The model under review builds one solid part; all positions refer to its coordinate system, in mm. A direction names the side the tool comes from. Coordinates: 2 decimals unless noted, no trailing zeros. Loops run counter-clockwise (first coordinate to the right, second up) from the corner with the lowest first, then second, coordinate; pieces in that order, holes last. Notation, with made-up numbers: M -17,51.25 L -13,51.25 A21 cw -13,63.25 Z; hole C 40.25,53 d7. An arc over 180 degrees is marked long. One line per item, written item: value.
```python
from build123d import *

# Parameters (mm, degrees)
F0_W      = 99.06
F0_H      = 99.06
F1_DEPTH  = 4.445
F0_W_2    = 101.6
F0_H_2    = 101.6
F2_DEPTH  = 63.5
F5_R      = 14.2875
F7_DEPTH  = 25.4
F3_R      = 14.2875
F3_R_2    = 13.193858
F8_DEPTH  = 25.4
F4_R      = 14.2875
F4_R_2    = 14.425909
F9_DEPTH  = 25.4
F6_R      = 14.2875
F10_DEPTH = 25.4
F11_R     = 14.2875
F12_DEPTH = 25.4


with BuildPart() as f1:
    # F0 (on Top) → F1 (new body)
    with BuildSketch(Plane.XY):
        Rectangle(F0_W, F0_H)
    extrude(amount=F1_DEPTH)

    # F0 (on Top) → F2 (join)
    with BuildSketch(Plane.XY):
        Rectangle(F0_W_2, F0_H_2)
        Rectangle(F0_W, F0_H, mode=Mode.SUBTRACT)
    extrude(amount=F2_DEPTH)

    # F5 (on face) → F7 (cut)
    with BuildSketch(Plane.XZ.offset(50.8)):
        with Locations((-27.728472, 33.152512)):
            Circle(F5_R)
        with Locations((26.523072, 33.849479)):
            Circle(F5_R)
    extrude(amount=-F7_DEPTH, mode=Mode.SUBTRACT)

    # F3 (on face) → F8 (cut)
    with BuildSketch(Plane.YZ.offset(50.8)):
        with Locations((-27.133925, 33.572733)):
            Circle(F3_R)
        with Locations((24.041634, 33.572733)):
            Circle(F3_R_2)
    extrude(amount=-F8_DEPTH, mode=Mode.SUBTRACT)

    # F4 (on face) → F9 (cut)
    with BuildSketch(Plane(origin=(0, 50.8, 0), x_dir=(-1, 0, 0), z_dir=(0, 1, 0))):
        with Locations((-27.319755, 33.915631)):
            Circle(F4_R)
        with Locations((28.376452, 33.915631)):
            Circle(F4_R_2)
    extrude(amount=F9_DEPTH, mode=Mode.SUBTRACT)

    # F6 (on face) → F10 (cut)
    with BuildSketch(Plane(origin=(-50.8, 0, 0), x_dir=(0, -1, 0), z_dir=(-1, 0, 0))):
        with Locations((-24.966941, 34.00825)):
            Circle(F6_R)
        with Locations((27.751417, 33.17856)):
            Circle(F6_R)
    extrude(amount=-F10_DEPTH, mode=Mode.SUBTRACT)

    # F11 (on face) → F12 (cut)
    with BuildSketch(Plane(origin=(0, 50.8, 0), x_dir=(-1, 0, 0), z_dir=(0, 1, 0))):
        with Locations((-25.37245, 35.114542)):
            Circle(F11_R)
        with Locations((23.656343, 35.114542)):
            Circle(F11_R)
    extrude(amount=-F12_DEPTH, mode=Mode.SUBTRACT)


solid = f1.part
```
(1) To check wall thickness, follow L1, parallel to X at y = -14, z = 44; L2, parallel to Z at x = -29, y = 30.5 (3 decimals). State the ranges of each line that lie inside material, in increasing order. Write a range as [from, to].
Checks:
L1: [-50.8, -49.53], [49.53, 50.8]
L2: [0, 4.445]
(2) Add section C-C on x = 34. State the section outline as (y, z) points (3 decimals).
Checks:
outline: M -50.8,0 L 50.8,0 L 50.8,23.726 L 49.53,23.726 L 49.53,4.445 L -49.53,4.445 L -49.53,21.675 L -50.8,21.675 Z; M -50.8,46.024 L -49.53,46.024 L -49.53,63.5 L -50.8,63.5 Z; M 49.53,46.503 L 50.8,46.503 L 50.8,63.5 L 49.53,63.5 Z
(3) Add section A-A on z = 56. State the section outline as (x, y) points, then the cut area to 3 significant figures.
Checks:
outline: M -50.8,-50.8 L 50.8,-50.8 L 50.8,50.8 L -50.8,50.8 Z; hole M -49.53,-49.53 L 49.53,-49.53 L 49.53,49.53 L -49.53,49.53 Z
area: 510 mm^2
(4) Insertion check: pin 1 Ø3 at (x, y) = (-30, 24) entering from +Z (3 decimals). The pin has a flat end and moves straight along its axis. Give the tip position at first contact, or say it passes through.
Checks:
pin 1: z = 4.445
(5) Add section D-D on y = -21. State the section outline as (x, z) points (3 decimals).
Checks:
outline: M -50.8,0 L 50.8,0 L 50.8,20.669 L 49.53,20.669 L 49.53,4.445 L -49.53,4.445 L -49.53,20.587 L -50.8,20.587 Z; M -50.8,45.77 L -49.53,45.77 L -49.53,63.5 L -50.8,63.5 Z; M 49.53,46.477 L 50.8,46.477 L 50.8,63.5 L 49.53,63.5 Z
(6) Draft analysis for pull direction X (two halves, no side actions). For faces 1 (the face through (35.903, 50.174, 44.771)), 2 (the face through (-50.17, -34.34, 20.5)), 3 (the face through (50.8, -1, 31)), state which applies: pulls with the +X half, pulls with the -X half, needs draft (parallel to the pull), parting line crosses it, or undercut.
Checks:
face 1: undercut
face 2: needs draft
face 3: pulls with the +X half
(7) Add section B-B on y = -2. State the section outline as (x, z) points (3 decimals), then the cut area to 3 significant figures.
Checks:
outline: M -50.8,0 L 50.8,0 L 50.8,63.5 L 49.53,63.5 L 49.53,4.445 L -49.53,4.445 L -49.53,63.5 L -50.8,63.5 Z
area: 602 mm^2
(8) Tool access review of faces 4 (the face through (-50.174, 36.305, 25.315)), 5 (the face through (50.174, -30.231, 19.625)), 6 (the face through (-1, 49.53, 34)), 7 (the face through (23.43, -50.17, 19.9)), 8 (the face through (-13.126, 50.174, 44.771)): name each direction out of +Z, -Z, +X, -X, +Y, -Y from which nothing blocks a thin tool from reaching the whole face with its end or side.
Checks:
face 4: -X
face 5: +X
face 6: +Z
face 7: -Y
face 8: +Y
